from build123d import *

# Parameters (mm, degrees)
F0_W     = 10
F0_H     = 10
F1_DEPTH = 10
F4_R     = 2.15
F3_R     = 2.5
F7_DEPTH = 25
F8_W     = 4.25
F8_H     = 1.8911467679
F9_DEPTH = 63
F10_R    = 1.5
F11_R    = 2


# Not quite as in the source:
# - an extrude ends at something that could not be found from the text; its depth is read off the source's solid


with BuildPart() as f1:
    # F0 (on Front) → F1 (new body, symmetric)
    with BuildSketch(Plane.XZ):
        Rectangle(F0_W, F0_H)
    extrude(amount=F1_DEPTH, both=True)

    # F5: sweep along a path in F2
    with BuildLine(Plane.XZ) as f5_path:
        Line((0, 0), (12.8993773854, 0))
        ThreePointArc((12.8993773854, 0), (14.6201066944, 0.5425438671), (15.7184552477, 1.97393957))
        Line((15.7184552477, 1.97393957), (20.1303021499, 14.0953893118))
    # F4 (on face) → F5 (sweep)
    with BuildSketch(Plane.YZ.offset(5)):
        Circle(F4_R)
    sweep(path=f5_path.line)

    # F6: F1 across plane


with BuildPart() as f1_1:
    add(f1.part)
    add(f1.part.mirror(Plane.YZ))

    # F3 (on face) → F7 (cut)
    with BuildSketch(Plane.XZ.offset(10)):
        Circle(F3_R)
    extrude(amount=-F7_DEPTH, mode=Mode.SUBTRACT)

    # F8 (on face) → F9 (cut, through all)
    with BuildSketch(Plane.XZ.offset(10)):
        with Locations((0.225, -5.9455733839)):
            Rectangle(F8_W, F8_H)
        with BuildLine():
            Line((-1.9, -1.6248076809), (-1.9, -5))
            Line((-1.9, -5), (2.35, -5))
            Line((2.35, -5), (2.35, -0.8529361055))
            ThreePointArc((2.35, -0.8529361055), (0.4467341852, -2.4597618925), (-1.9, -1.6248076809))
        make_face()
        with BuildLine():
            Line((-1.9, 0), (-1.9, -1.6248076809))
            ThreePointArc((-1.9, -1.6248076809), (0.4467341852, -2.4597618925), (2.35, -0.8529361055))
            Line((2.35, -0.8529361055), (2.35, 0))
            Line((2.35, 0), (-1.9, 0))
        make_face()
    extrude(amount=-F9_DEPTH, mode=Mode.SUBTRACT)

    # F10
    f10_edges = [f1_1.edges().sort_by_distance(p)[0] for p in [
        (5, 0, 5),
        (-5, 0, 5),
        (5, 0, -5),
        (-5, 0, -5),
    ]]
    fillet(f10_edges, radius=F10_R)

    # F11
    f11_edges = [f1_1.edges().sort_by_distance(p)[0] for p in [
        (-20.130302, -2.15, 14.095389),
        (20.130302, -2.15, 14.095389),
    ]]
    fillet(f11_edges, radius=F11_R)


solid = f1_1.part
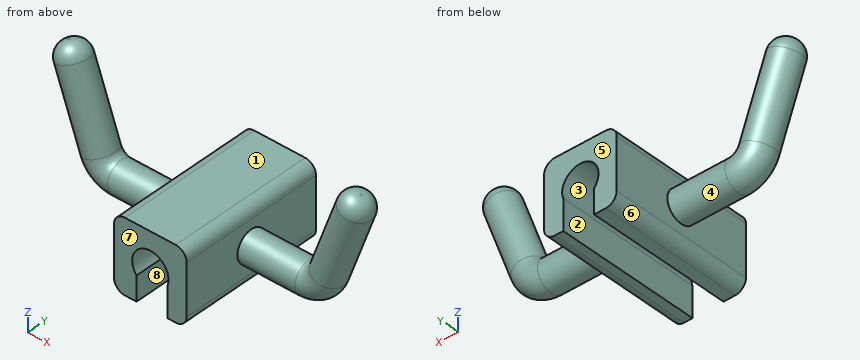
Geometry: final body of the model. Coordinates: model frame, mm. Face numbers are marked on the shaded views. A direction names the side the tool comes from. Round coordinates to 2 decimals unless told otherwise and drop trailing zeros. Loops run counter-clockwise (first coordinate to the right, second up) from the corner with the lowest first, then second, coordinate; pieces in that order, holes last. Notation, with made-up numbers: (-35.75, 30) -> (-17.75, 30) arc R28 cw to (-17.75, 57) -> close; hole circle Ø7 at (84, 33). An arc over 180 degrees is marked (long way). One line per question, with ' | ' between items. Start each with the question number.
1. Line query: line 1 along X through (y, z) = (4.75, 0); line 2 along X through (y, z) = (-1, 4); line 3 along Z through (x, y) = (0, -6). Output: solid intervals per line, ascending. Write a range as [from, to].
2. Set-up query: the marked faces 1, 2, 3, 4 and 5. Return all of +Z, -Z, +X, -X, +Y, -Y with unobstructed straight access to the full face (end or side cutting, diameter ignored); none if empty.
3. Section C-C on z = 4.5. Count the separate pieces of the cut face and the enclosed holes in it, and give its area (3 significant figures).
4. Mould query, pull axis X, two halves, no side actions, for the marked faces 6, 7 and 8. Classes: pulls with the +X half, pulls with the -X half, needs draft (parallel to the pull), parting line crosses it, or undercut.
5. Section B-B on x = 0. Output: boundary loops of the cut face in (y, z), and give its area (3 significant figures).
6. Section A-A on y = -8.25. Output: boundary loops of the cut face in (x, z), and give its area (3 significant figures).
7. Contact query for flat-ended pins moving along their axis: pin 1 (6 mm diameter, centred on x = -13, z = 1.5, fed in from -Y); pin 2 (12 mm diameter, centred on x = -10, y = -6, fed in from +Z); pin 3 (2.5 mm diameter, centred on y = -5, z = -4, fed in from +X); pin 4 (4 mm diameter, centred on x = -6, z = 7.5, fed in from +Y). Output: stop coordinate, or through.
8. Section D-D on x = 8.5. Output: boundary loops of the cut face in (y, z), and give its area (3 significant figures).
Returned:
1) line 1: x = [-5, -2.5], [2.5, 5] | line 2: x = [-18.48, -14.43], [-4.91, 4.91], [14.43, 18.48] | line 3: z = [2.5, 5]
2) face 1: +Z, +Y, -Y | face 2: -Z, +Y, -Y | face 3: +Y, -Y | face 4: none | face 5: +Z, -Z, +X, -X, +Y
3) separate pieces: 3 | enclosed holes: 0 | area: 216 mm2
4) face 6: pulls with the -X half | face 7: needs draft | face 8: undercut
5) outline: (-10, 2.5) -> (10, 2.5) -> (10, 5) -> (-10, 5) -> close | area: 50.0 mm2
6) outline: (-5, -3.5) arc R1.5 ccw to (-3.5, -5) -> (-1.9, -5) -> (-1.9, -1.62) arc R2.5 cw (long way) to (2.35, -0.85) -> (2.35, -5) -> (3.5, -5) arc R1.5 ccw to (5, -3.5) -> (5, 3.5) arc R1.5 ccw to (3.5, 5) -> (-3.5, 5) arc R1.5 ccw to (-5, 3.5) -> close | area: 66.2 mm2
7) pin 1: stops at y = -2.15 | pin 2: stops at z = 4.91 | pin 3: stops at x = 5 | pin 4: passes through
8) outline: circle Ø4.3 at (0, 0) | area: 14.5 mm2
